```python
from build123d import *

# Parameters (mm, degrees)
F1_DEPTH = 4
F2_R     = 2.5
F2_R_2   = 10.2663789445
F2_R_3   = 5.2288220919
F3_DEPTH = 4
F5_R     = 2.5
F5_R_2   = 10.2663789445
F5_R_3   = 5.2288220919
F6_DEPTH = 4


with BuildPart() as f1:
    # F0 (on Front) → F1 (new body)
    with BuildSketch(Plane.XZ):
        with BuildLine():
            Line((9.2053477168, 40), (5.1, 40))
            ThreePointArc((5.1, 40), (0, 34.9), (-5.1, 40))
            Line((-5.1, 40), (-9.2053477168, 40))
            ThreePointArc((-9.2053477168, 40), (-9.7179108497, 38.7625631329), (-10.9553477168, 38.25))
            Line((-10.9553477168, 38.25), (-16, 38.25))
            ThreePointArc((-16, 38.25), (-17.2374368671, 38.7625631329), (-17.75, 40))
            Line((-17.75, 40), (-20, 40))
            Line((-20, 40), (-20, 20))
            Line((-20, 20), (20, 20))
            Line((20, 20), (20, 40))
            Line((20, 40), (17.75, 40))
            ThreePointArc((17.75, 40), (17.2374368671, 38.7625631329), (16, 38.25))
            Line((16, 38.25), (10.9553477168, 38.25))
            ThreePointArc((10.9553477168, 38.25), (9.7179108497, 38.7625631329), (9.2053477168, 40))
        make_face()
        with BuildLine():
            Line((1.75, 29.0446522832), (1.75, 24))
            ThreePointArc((1.75, 24), (0, 22.25), (-1.75, 24))
            Line((-1.75, 24), (-1.75, 29.0446522832))
            ThreePointArc((-1.75, 29.0446522832), (0, 30.7946522832), (1.75, 29.0446522832))
        make_face(mode=Mode.SUBTRACT)
        with BuildLine():
            ThreePointArc((-5.1, 40), (0, 45.1), (5.1, 40))
            Line((5.1, 40), (9.2053477168, 40))
            ThreePointArc((9.2053477168, 40), (9.7179108497, 41.2374368671), (10.9553477168, 41.75))
            Line((10.9553477168, 41.75), (16, 41.75))
            ThreePointArc((16, 41.75), (17.2374368671, 41.2374368671), (17.75, 40))
            Line((17.75, 40), (20, 40))
            Line((20, 40), (20, 60))
            Line((20, 60), (-20, 60))
            Line((-20, 60), (-20, 40))
            Line((-20, 40), (-17.75, 40))
            ThreePointArc((-17.75, 40), (-17.2374368671, 41.2374368671), (-16, 41.75))
            Line((-16, 41.75), (-10.9553477168, 41.75))
            ThreePointArc((-10.9553477168, 41.75), (-9.7179108497, 41.2374368671), (-9.2053477168, 40))
            Line((-9.2053477168, 40), (-5.1, 40))
        make_face()
        with BuildLine():
            ThreePointArc((1.75, 50.9553477168), (0, 49.2053477168), (-1.75, 50.9553477168))
            Line((-1.75, 50.9553477168), (-1.75, 56))
            ThreePointArc((-1.75, 56), (0, 57.75), (1.75, 56))
            Line((1.75, 56), (1.75, 50.9553477168))
        make_face(mode=Mode.SUBTRACT)
    extrude(amount=F1_DEPTH)

    # F2 (on face) → F3 (join)
    with BuildSketch(Plane.YZ.offset(20)):
        with BuildLine():
            Line((-32.3069637418, 0), (-5, 0))
            ThreePointArc((-5, 0), (-1.4644660941, 1.4644660941), (0, 5))
            Line((0, 5), (0, 60))
            Line((0, 60), (-4, 60))
            Line((-4, 60), (-36.3334842795, 16.0803529313))
            ThreePointArc((-36.3334842795, 16.0803529313), (-37.0573638664, 14.6760747904), (-37.3069637418, 13.1160431703))
            Line((-37.3069637418, 13.1160431703), (-37.3069637418, 5))
            ThreePointArc((-37.3069637418, 5), (-35.8424976477, 1.4644660941), (-32.3069637418, 0))
        make_face()
        with Locations((-32.3069637418, 5)):
            Circle(F2_R, mode=Mode.SUBTRACT)
        with Locations((-5, 5)):
            Circle(F2_R, mode=Mode.SUBTRACT)
        with Locations((-17.2130409628, 17.1549171209)):
            Circle(F2_R_2, mode=Mode.SUBTRACT)
        with Locations((-9.977567941, 35.5724841356)):
            Circle(F2_R_3, mode=Mode.SUBTRACT)
    extrude(amount=F3_DEPTH)

    # F5 (on 3pt) → F6 (join)
    with BuildSketch(Plane.YZ.offset(-20)):
        with BuildLine():
            Line((-32.3069637418, 0), (-5, 0))
            ThreePointArc((-5, 0), (-1.4644660941, 1.4644660941), (0, 5))
            Line((0, 5), (0, 60))
            Line((0, 60), (-4, 60))
            Line((-4, 60), (-24.0229353611, 32.8021809608))
            Line((-24.0229353611, 32.8021809608), (-36.3334842795, 16.0803529313))
            ThreePointArc((-36.3334842795, 16.0803529313), (-37.0573638664, 14.6760747904), (-37.3069637418, 13.1160431703))
            Line((-37.3069637418, 13.1160431703), (-37.3069637418, 5))
            ThreePointArc((-37.3069637418, 5), (-35.8424976477, 1.4644660941), (-32.3069637418, 0))
        make_face()
        with Locations((-32.3069637418, 5)):
            Circle(F5_R, mode=Mode.SUBTRACT)
        with Locations((-5, 5)):
            Circle(F5_R, mode=Mode.SUBTRACT)
        with Locations((-17.2130409628, 17.1549171209)):
            Circle(F5_R_2, mode=Mode.SUBTRACT)
        with Locations((-9.977567941, 35.5724841356)):
            Circle(F5_R_3, mode=Mode.SUBTRACT)
    extrude(amount=-F6_DEPTH)


solid = f1.part
```
Model file for the job. Use its own axes, mm. A direction names the side the tool comes from. Give positions to 0.01 mm unless a question says otherwise; leave off trailing zeros. Loops run counter-clockwise (first coordinate to the right, second up) from the corner with the lowest first, then second, coordinate; pieces in that order, holes last. Notation, with made-up numbers: (-0.5, 46.25) -> (30.5, 46.25) arc R8 cw to (30.5, 53.25) -> close; hole circle Ø9 at (-0.5, 64). An arc over 180 degrees is marked (long way). Use CSV: the item, a comma, the result in double quotes. Start each with the question number.
1) Tool access for faces 1 (the cylindrical face through (21.972, -2.615, 5.751)), 2 (the flat face through (0, -2, 20)), 3 (the flat face through (1.75, -2, 27)): list every direction of +Z, -Z, +X, -X, +Y, -Y with a clear straight run to the whole face (end or side of a thin tool).
2) Mould opens along Z. For faces 4 (the flat face through (21.97, -19.94, 38.35)), 5 (the cylindrical face through (0.04, -1.97, 22.25)), 6 (the flat face through (-22, -37.307, 9)) say: released by +Z, released by -Z, zero draft, split by the parting line, or undercut.
3) Slice it at C-C on y = -6. Give the cut face in (x, z).
4) Slice it at B-B on z = 44. Give the cut face in (x, y).
5) Slice it at A-A on x = 0. Give the cut face in (y, z), plus the area to 3 significant figures.
6) Flat gauge pins, fed straight in: pin 1 Ø9.5 at (y, z) = (-9.98, 35.57) entering from +X; pin 2 Ø2 at (x, y) = (12.5, -2) entering from -Z; pin 3 Ø12 at (x, z) = (6, 30.5) entering from -Y. Where does each tip first touch, or does it go through?
7) Wall check: line 1 (Z direction, x = 0, y = -1.55); line 2 (X direction, y = -22.5, z = 4.5); line 3 (Y direction, x = 10, z = 38). Give the ranges that are in metal, low to high.
8) Slice it at D-D on x = -21. Give the cut face in (y, z), plus the area to 3 significant figures.
Computed values:
1,face 1,"+X, -X"
1,face 2,"-Z, +Y, -Y"
1,face 3,"+Y, -Y"
2,face 4,"released by +Z"
2,face 5,"undercut"
2,face 6,"zero draft"
3,outline,"(-24, 0) -> (-20, 0) -> (-20, 2.71) -> (-24, 2.71) -> close; (-24, 7.29) -> (-20, 7.29) -> (-20, 32.18) -> (-24, 32.18) -> close; (-24, 38.97) -> (-20, 38.97) -> (-20, 57.28) -> (-24, 57.28) -> close; (20, 0) -> (24, 0) -> (24, 2.71) -> (20, 2.71) -> close; (20, 7.29) -> (24, 7.29) -> (24, 32.18) -> (20, 32.18) -> close; (20, 38.97) -> (24, 38.97) -> (24, 57.28) -> (20, 57.28) -> close"
4,outline,"(-24, -15.78) -> (-20, -15.78) -> (-20, -4) -> (-3.16, -4) -> (-3.16, 0) -> (-24, 0) -> close; (3.16, -4) -> (20, -4) -> (20, -15.78) -> (24, -15.78) -> (24, 0) -> (3.16, 0) -> close"
5,outline,"(-4, 20) -> (0, 20) -> (0, 22.25) -> (-4, 22.25) -> close; (-4, 30.79) -> (0, 30.79) -> (0, 34.9) -> (-4, 34.9) -> close; (-4, 45.1) -> (0, 45.1) -> (0, 49.21) -> (-4, 49.21) -> close; (-4, 57.75) -> (0, 57.75) -> (0, 60) -> (-4, 60) -> close"
5,area,"50.8 mm^2"
6,pin 1,"passes through"
6,pin 2,"stops at z = 20"
6,pin 3,"stops at y = -4"
7,line 1,"z = 20 to 22.25, 30.79 to 34.9, 45.1 to 49.21, 57.75 to 60"
7,line 2,"x = -24 to -20, 20 to 24"
7,line 3,"y = -4 to 0"
8,outline,"(-37.31, 5) arc R5 ccw to (-32.31, 0) -> (-5, 0) arc R5 ccw to (0, 5) -> (0, 60) -> (-4, 60) -> (-36.33, 16.08) arc R5 ccw to (-37.31, 13.12) -> close; hole circle Ø5 at (-32.31, 5); hole circle Ø20.53 at (-17.21, 17.15); hole circle Ø10.46 at (-9.98, 35.57); hole circle Ø5 at (-5, 5)"
8,area,"1,020 mm^2"
